Geometry: final body of the model. Coordinates: model frame, mm. Coordinates: 2 decimals unless noted, no trailing zeros. Write each loop counter-clockwise with the first axis right and the second up, starting at its lowest first coordinate (ties: lowest second). Pieces come first, ordered by that corner, then holes.
from build123d import *

# Parameters (mm, degrees)
SKETCH1_W           = 51
SKETCH1_H           = 71
BOSS_EXTRUDE1_DEPTH = 3
SKETCH2_W           = 4
SKETCH2_H           = 20
BOSS_EXTRUDE3_DEPTH = 3
SKETCH4_W           = 3.2
SKETCH4_H           = 20.5
CUT_EXTRUDE1_DEPTH  = 5
FILLET1_RADIUS      = 1.5
FILLET1_LENGTH      = 25.25
FILLET2_RADIUS      = 1.5
FILLET2_LENGTH      = 20.5
FILLET3_RADIUS      = 1.5
FILLET3_LENGTH      = 25.25


with BuildPart() as part:
    # Sketch1 → Boss-Extrude1 (new body)
    with BuildSketch(Plane(origin=(0, 0, 0), x_dir=(1, 0, 0), z_dir=(0, 1, 0))):
        Rectangle(SKETCH1_W, SKETCH1_H)
    extrude(amount=BOSS_EXTRUDE1_DEPTH)

    # Sketch2 → Boss-Extrude3 (add)
    with BuildSketch(Plane(origin=(0, 3, 0), x_dir=(1, 0, 0), z_dir=(0, 1, 0))):
        with Locations((-19.5, 0)):
            Rectangle(SKETCH2_W, SKETCH2_H)
    extrude(amount=BOSS_EXTRUDE3_DEPTH)

    # Sketch4 → Cut-Extrude1 (cut)
    with BuildSketch(Plane(origin=(0, 3, 0), x_dir=(1, 0, 0), z_dir=(0, 1, 0))):
        with Locations((23.9, 0)):
            Rectangle(SKETCH4_W, SKETCH4_H)
    extrude(amount=-CUT_EXTRUDE1_DEPTH, mode=Mode.SUBTRACT)

    # Sketch6 → Cut-Revolve1 (revolve, cut)
    with BuildSketch(Plane.XY.offset(-10.25)):
        with BuildLine():
            Line((22.90000003, 1.5), (24.89999997, 1.5))
            ThreePointArc((24.89999997, 1.5), (23.9, 0.50000003), (22.90000003, 1.5))
        make_face()
    cut_revolve1 = revolve(axis=Axis((22.90000003, 1.5, -10.25), (1, 0, 0)), mode=Mode.SUBTRACT)

    # Mirror1: Cut-Revolve1 across plane
    add(cut_revolve1.mirror(Plane.XY), mode=Mode.SUBTRACT)

    # Fillet1: full round fillet: the end face becomes a half cylinder, R = half its width
    fillet1_face = Plane((25.5, 1.5, 22.875), x_dir=(0, 0, 1), z_dir=(1, 0, 0))  # on the end face: x along it, z out of the body
    fillet1_slab = fillet1_face.offset(-FILLET1_RADIUS / 2) * Box(FILLET1_LENGTH, 2 * FILLET1_RADIUS, FILLET1_RADIUS, mode=Mode.PRIVATE)  # the body's end, R deep
    fillet1_round = Plane((24, 1.5, 22.875), x_dir=(1, 0, 0), z_dir=(0, 0, 1)) * Cylinder(FILLET1_RADIUS, FILLET1_LENGTH, mode=Mode.PRIVATE)  # its axis R under the face
    add(fillet1_slab - fillet1_round, mode=Mode.SUBTRACT)

    # Fillet2: full round fillet: the end face becomes a half cylinder, R = half its width
    fillet2_face = Plane((22.3, 1.5, 0), x_dir=(0, 0, -1), z_dir=(1, 0, 0))  # on the end face: x along it, z out of the body
    fillet2_slab = fillet2_face.offset(-FILLET2_RADIUS / 2) * Box(FILLET2_LENGTH, 2 * FILLET2_RADIUS, FILLET2_RADIUS, mode=Mode.PRIVATE)  # the body's end, R deep
    fillet2_round = Plane((20.8, 1.5, 0), x_dir=(1, 0, 0), z_dir=(0, 0, -1)) * Cylinder(FILLET2_RADIUS, FILLET2_LENGTH, mode=Mode.PRIVATE)  # its axis R under the face
    add(fillet2_slab - fillet2_round, mode=Mode.SUBTRACT)

    # Fillet3: full round fillet: the end face becomes a half cylinder, R = half its width
    fillet3_face = Plane((25.5, 1.5, -22.875), x_dir=(0, 0, -1), z_dir=(1, 0, 0))  # on the end face: x along it, z out of the body
    fillet3_slab = fillet3_face.offset(-FILLET3_RADIUS / 2) * Box(FILLET3_LENGTH, 2 * FILLET3_RADIUS, FILLET3_RADIUS, mode=Mode.PRIVATE)  # the body's end, R deep
    fillet3_round = Plane((24, 1.5, -22.875), x_dir=(1, 0, 0), z_dir=(0, 0, -1)) * Cylinder(FILLET3_RADIUS, FILLET3_LENGTH, mode=Mode.PRIVATE)  # its axis R under the face
    add(fillet3_slab - fillet3_round, mode=Mode.SUBTRACT)


solid = part.part
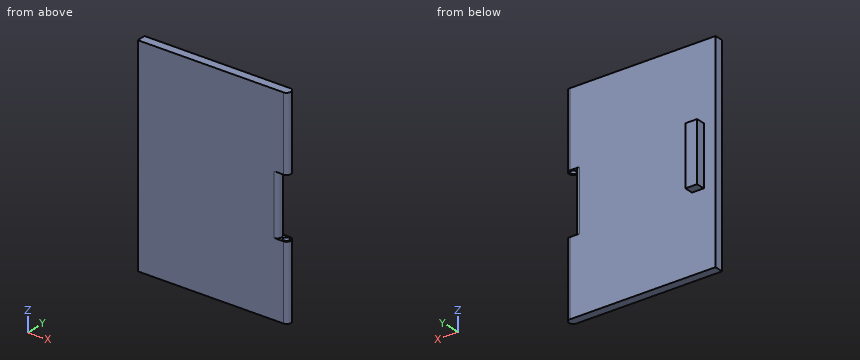
Item 1: Pin query (flat end, axial travel): pin 1 (3.5 mm diameter, centred on y = 5, z = 1, fed in from +X); pin 2 (0.9 mm diameter, centred on x = -18.5, y = 4.5, fed in from -Z); pin 3 (12 mm diameter, centred on x = -5.5, z = 25.5, fed in from +Y). Return the tip coordinate at first contact, or that it passes through.
Derived:
pin 1: stops at x = -17.5
pin 2: stops at z = -10
pin 3: stops at y = 3
Item 2: Section C-C, the plane x = -10. Output: boundary loops of the cut face in (y, z).
Derived:
outline: (0, -35.5) - (3, -35.5) - (3, 35.5) - (0, 35.5) - close
Item 3: Material intervals for probe 1 along Y at (x, z) = (-12, -5.5); probe 2 along X at (y, z) = (1.3, 21.5); probe 3 along X at (y, z) = (2.7, -15), sorted ascending.
Derived:
probe 1: y = 0 to 3
probe 2: x = -25.5 to 25.49
probe 3: x = -25.5 to 24.9
Item 4: Section B-B, the plane z = 27. Output: boundary loops of the cut face in (x, y), plus the area to 3 significant figures.
Derived:
outline: (-25.5, 0) - (24, 0) arc R1.5 ccw to (24, 3) - (-25.5, 3) - close
area: 152 mm2
Item 5: Section A-A, the plane y = 1.5. Output: boundary loops of the cut face in (x, z), plus the area to 3 significant figures.
Derived:
outline: (-25.5, -35.5) - (25.5, -35.5) - (25.5, -10.25) - (24.9, -10.25) arc R1 cw to (22.9, -10.25) - (22.3, -10.25) - (22.3, 10.25) - (22.9, 10.25) arc R1 cw to (24.9, 10.25) - (25.5, 10.25) - (25.5, 35.5) - (-25.5, 35.5) - close
area: 3,550 mm2
